Geometry check sheet. Reference: drawing and pictorial views, mm from the part's lowest x, y, z. Coordinates: 2 decimals unless noted, no trailing zeros. Order: outer loops, then holes, each group sorted by start corner. A loop starts at its lowest first (then second) coordinate and runs counter-clockwise, first axis right, second up. Notation, with made-up numbers: (53.5, -30) -> (97.5, -30) arc R18 ccw to (97.5, 4) -> close; hole circle Ø10 at (-30, -19.5). An arc over 180 degrees is marked (long way). Use CSV: the item, a comma, the result in double quotes. Start each with the question number.
1) Sectioned sample at B-B on x = 37. Record the boundary of the cut face in (y, z).
2) Scan lines: line 1 along Z through (x, y) = (28.5, 7); line 2 along Z through (x, y) = (86.5, 12.25); line 3 along X through (y, z) = (5.5, 179) (1 decimal). Record each from-to range of solid material in increasing order.
3) Go/stop test with a flat-tipped pin: pin 1 (6 mm diameter, centred on x = 88.5, y = 15, fed in from +Z). Record where the tip stops, or that it passes through.
4) Sectioned sample at C-C on z = 150. Record the boundary of the cut face in (x, y), then the cut area to 3 significant figures.
5) Sectioned sample at A-A on y = 17. Record the boundary of the cut face in (x, z).
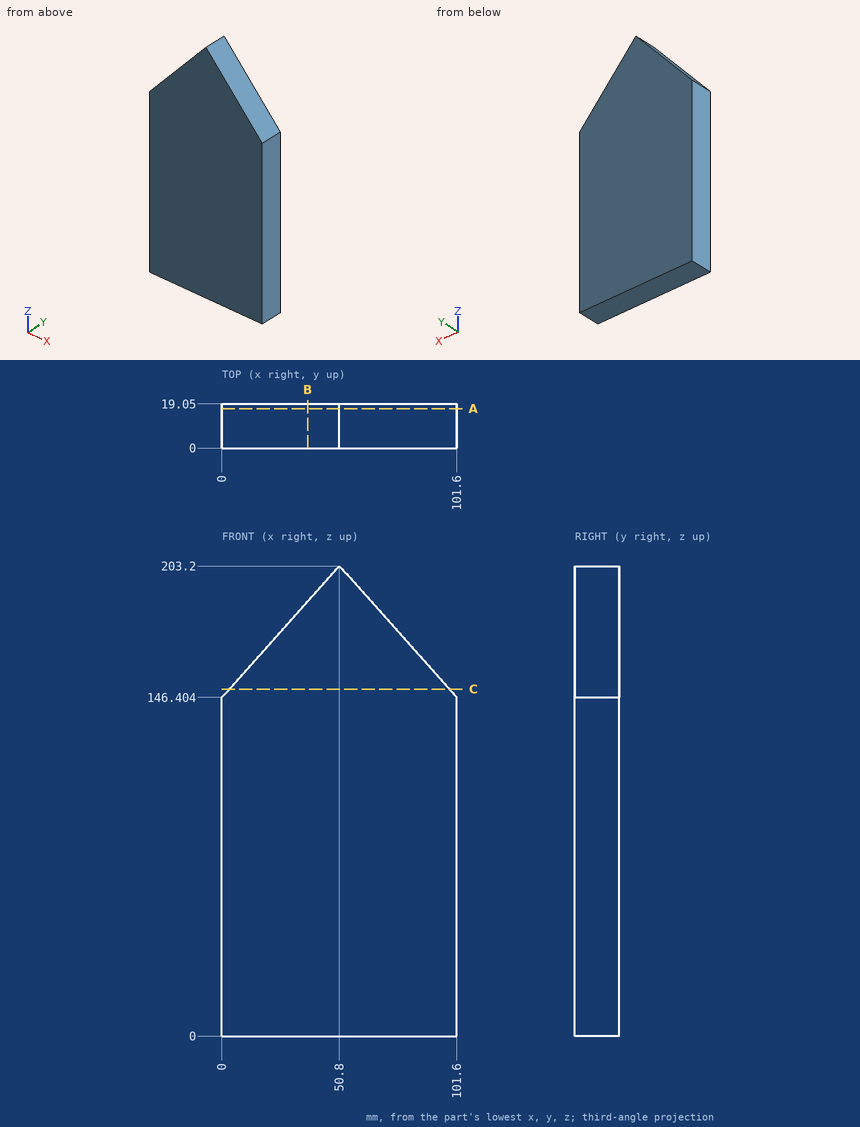
Answers follow:
1,outline,"(0, 0) -> (19.05, 0) -> (19.05, 187.77) -> (0, 187.77) -> close"
2,line 1,"z = 0 to 178.27"
2,line 2,"z = 0 to 163.29"
2,line 3,"x = 29.2 to 72.4"
3,pin 1,"stops at z = 164.4"
4,outline,"(3.22, 0) -> (98.38, 0) -> (98.38, 19.05) -> (3.22, 19.05) -> close"
4,area,"1,810 mm²"
5,outline,"(0, 0) -> (101.6, 0) -> (101.6, 146.4) -> (50.8, 203.2) -> (0, 146.4) -> close"
